Source: CAD feature listing. Evaluate the final solid. Frame: model axes, mm. A direction names the side the tool comes from. Coordinates: 2 decimals unless noted, no trailing zeros. Write each loop counter-clockwise with the first axis right and the second up, starting at its lowest first coordinate (ties: lowest second). Pieces come first, ordered by that corner, then holes. Notation, with made-up numbers: M 16.25,30.5 L 74.25,30.5 A35 ccw 74.25,64.5 Z; hole C 75.5,50.5 d11. An arc over 180 degrees is marked long. One line per item, written item: value. Start each with the question number.
Item 1: Cut plane D-D, the plane y = -34. Output: boundary loops of the cut face in (x, z), then the cut area to 3 significant figures.
Item 2: Pin query (flat end, axial travel): P1, Ø11, axis at y = 24, z = 10.5, coming from the -X side; P2, Ø4, axis at x = -12, z = 21.5, coming from the -Y side; P3, Ø4, axis at x = 11.5, z = 26.5, coming from the +Y side; P4, Ø4, axis at x = 12, z = 27, coming from the -Y side. Return the tip coordinate at first contact, or that it passes through.
Item 3: Cut plane B-B, the plane z = 11.5. Output: boundary loops of the cut face in (x, y), then the cut area to 3 significant figures.
Item 4: Ray query, L1, parallel to X at y = 16, z = 11.5; L2, parallel to Y at x = -15, z = 10; L3, parallel to X at y = -25.5, z = 23. Return the intervals inside material, ascending. Write a range as from..to.
Item 5: Set-up query: faces 4 (the flat face through (-14, 31, 29)), 5 (the flat face through (13.4, -24, 9)), 6 (the cylindrical face through (-15.479, 28.795, 8.722)), 7 (the flat face through (14, 31, 29)), 8 (the cylindrical face through (0.126, -0.744, 5.008)). Return all of +Z, -Z, +X, -X, +Y, -Y with unobstructed straight access to the full face (end or side cutting, diameter ignored); none if empty.
Item 6: Cut plane A-A, the plane x = 15. Output: boundary loops of the cut face in (y, z).
Item 7: Mould query, pull axis Y, two halves, no side actions, for faces 1 (the flat face through (17.5, -1, 10)), 2 (the flat face through (0, -40, 25)), 3 (the flat face through (-12, 22, 25)). Classes: released by +Y, released by -Y, zero draft, split by the parting line, or undercut.
Item 8: Cut plane C-C, the plane z = 32.5. Output: boundary loops of the cut face in (x, y), then the cut area to 3 significant figures.
```python
from build123d import *

# Parameters (mm, degrees)
F0_W      = 35
F0_H      = 95
F1_DEPTH  = 20
F2_W      = 5
F2_H      = 18
F2_W_2    = 18
F3_DEPTH  = 10
F6_DEPTH  = 28
F8_DEPTH  = 9
F9_R      = 3
F10_R     = 5.05
F11_DEPTH = 4.1
F12_R     = 5.05
F13_DEPTH = 4.1


with BuildPart() as f1:
    # F0 (on Top) → F1 (new body)
    with BuildSketch(Plane.XY):
        Rectangle(F0_W, F0_H)
    extrude(amount=F1_DEPTH)

    # F2 (on face) → F3 (join)
    with BuildSketch(Plane.XY.offset(20)):
        with Locations((-11.5, -31)):
            Rectangle(F2_W, F2_H)
        with Locations((11.5, -31)):
            Rectangle(F2_W, F2_H)
        with Locations((11.5, 31)):
            Rectangle(F2_W, F2_H)
        with Locations((-11.5, 31)):
            Rectangle(F2_W, F2_H)
        with Locations((0, -31)):
            Rectangle(F2_W_2, F2_H)
        with Locations((0, 31)):
            Rectangle(F2_W_2, F2_H)
    extrude(amount=F3_DEPTH)

    # F5 (on face) + F4 (on face) → F6 (join)
    with BuildSketch(Plane.YZ.offset(14)):
        with BuildLine():
            Line((-40, 30), (-22, 30))
            ThreePointArc((-22, 30), (-31, 39), (-40, 30))
        make_face()
    with BuildSketch(Plane.YZ.offset(14)):
        with BuildLine():
            Line((22, 30), (40, 30))
            ThreePointArc((40, 30), (31, 39), (22, 30))
        make_face()
    extrude(amount=-F6_DEPTH)

    # F7 (on Right) → F8 (cut, symmetric)
    with BuildSketch(Plane.YZ):
        with BuildLine():
            ThreePointArc((7.6e-09, 76), (-25.1022907294, 65.6022907348), (-35.5, 40.5))
            Line((-35.5, 40.5), (35.5, 40.5))
            ThreePointArc((35.5, 40.5), (25.1022907348, 65.6022907294), (7.6e-09, 76))
        make_face()
        with BuildLine():
            Line((-35.5, 76), (-35.5, 40.5))
            ThreePointArc((-35.5, 40.5), (-25.1022907294, 65.6022907348), (7.6e-09, 76))
            Line((7.6e-09, 76), (-35.5, 76))
        make_face()
        with BuildLine():
            ThreePointArc((7.6e-09, 76), (25.1022907348, 65.6022907294), (35.5, 40.5))
            Line((35.5, 40.5), (35.5, 76))
            Line((35.5, 76), (7.6e-09, 76))
        make_face()
        with BuildLine():
            Line((35.5, 40.5), (-35.5, 40.5))
            ThreePointArc((-35.5, 40.5), (0, 5), (35.5, 40.5))
        make_face()
    extrude(amount=F8_DEPTH, both=True, mode=Mode.SUBTRACT)

    # F9
    f9_edges = [f1.edges().sort_by_distance(p)[0] for p in [
        (0, -47.5, 20),
        (0, 47.5, 20),
    ]]
    fillet(f9_edges, radius=F9_R)

    # F10 (on face) → F11 (cut)
    with BuildSketch(Plane.YZ.offset(17.5)):
        with Locations((-23.8, 8.45)):
            Circle(F10_R)
        with Locations((23.8, 8.45)):
            Circle(F10_R)
    extrude(amount=-F11_DEPTH, mode=Mode.SUBTRACT)

    # F12 (on face) → F13 (cut)
    with BuildSketch(Plane(origin=(-17.5, 0, 0), x_dir=(0, -1, 0), z_dir=(-1, 0, 0))):
        with Locations((-23.75, 8.5)):
            Circle(F12_R)
        with Locations((23.75, 8.5)):
            Circle(F12_R)
    extrude(amount=-F13_DEPTH, mode=Mode.SUBTRACT)


solid = f1.part
```
From the geometry:
1. outline: M -17.5,0 L 17.5,0 L 17.5,20 L 14,20 L 14,38.49 L 9,38.49 L 9,30.29 L -9,30.29 L -9,38.49 L -14,38.49 L -14,20 L -17.5,20 Z
1. area: 1,070 mm²
2. P1: stops at x = -17.5
2. P2: stops at y = -46.16
2. P3: stops at y = 40
2. P4: stops at y = -40
3. outline: M -17.5,-47.5 L 17.5,-47.5 L 17.5,-27.82 L 13.4,-27.82 L 13.4,-19.78 L 17.5,-19.78 L 17.5,19.78 L 13.4,19.78 L 13.4,27.82 L 17.5,27.82 L 17.5,47.5 L -17.5,47.5 L -17.5,27.81 L -13.4,27.81 L -13.4,19.69 L -17.5,19.69 L -17.5,-19.69 L -13.4,-19.69 L -13.4,-27.81 L -17.5,-27.81 Z; hole M -9,-20.48 L 9,-20.48 L 9,20.48 L -9,20.48 Z
3. area: 2,460 mm²
4. L1: x = -17.5..-9, 9..17.5
4. L2: y = -47.5..-28.57, -18.93..18.93, 28.57..47.5
4. L3: x = -14..-9, 9..14
5. face 4: +Z, -X, +Y, -Y
5. face 5: +X
5. face 6: -X
5. face 7: +Z, +X, +Y, -Y
5. face 8: +Z
6. outline: M -47.5,0 L 47.5,0 L 47.5,17 A3 ccw 44.5,20 L -44.5,20 A3 ccw -47.5,17 Z; hole C -23.8,8.45 d10.1; hole C 23.8,8.45 d10.1
7. face 1: zero draft
7. face 2: released by -Y
7. face 3: undercut
8. outline: M -14,-39.65 L 14,-39.65 L 14,-22.35 L 9,-22.35 L 9,-34.59 L -9,-34.59 L -9,-22.35 L -14,-22.35 Z; M -14,22.35 L -9,22.35 L -9,34.59 L 9,34.59 L 9,22.35 L 14,22.35 L 14,39.65 L -14,39.65 Z
8. area: 528 mm²
